Work out the finished part from the listing and answer in its coordinate system (mm). A direction names the side the tool comes from. Coordinates: 2 decimals unless noted, no trailing zeros. Loops run counter-clockwise (first coordinate to the right, second up) from the corner with the lowest first, then second, coordinate; pieces in that order, holes last. Notation, with made-up numbers: (86.25, 81.5) -> (129.25, 81.5) arc R20 ccw to (129.25, 110.5) -> close; hole circle Ø4 at (67.25, 19). An arc over 180 degrees is marked (long way). Use a Markdown table: item, result. Add a question column.
```python
from build123d import *

# Parameters (mm, degrees)
SKETCH_R     = 11.5
SKETCH_R_2   = 1.3
PAD_DEPTH    = 3
POCKET_DEPTH = 1.4


with BuildPart() as part:
    # Sketch → Pad (new body)
    with BuildSketch(Plane.XY):
        with BuildLine():
            ThreePointArc((13.066667, 5.026154), (0, 14), (-13.066667, 5.026154))
            ThreePointArc((-17.230769, 2.485461), (-14.71661, 3.047599), (-13.066667, 5.026154))
            ThreePointArc((-17.230769, 2.485461), (-20, 0), (-17.230769, -2.485461))
            ThreePointArc((-13.066667, -5.026154), (-14.71661, -3.047599), (-17.230769, -2.485461))
            ThreePointArc((-13.066667, -5.026154), (0, -14), (13.066667, -5.026154))
            ThreePointArc((17.230769, -2.485461), (14.71661, -3.047599), (13.066667, -5.026154))
            ThreePointArc((17.230769, -2.485461), (20, 0), (17.230769, 2.485461))
            ThreePointArc((13.066667, 5.026154), (14.71661, 3.047599), (17.230769, 2.485461))
        make_face()
        Circle(SKETCH_R, mode=Mode.SUBTRACT)
        with Locations((-17.5, 0)):
            Circle(SKETCH_R_2, mode=Mode.SUBTRACT)
        with Locations((17.5, 0)):
            Circle(SKETCH_R_2, mode=Mode.SUBTRACT)
    extrude(amount=PAD_DEPTH)

    # Sketch001 (on Face13 of Pad) → Pocket (cut)
    with BuildSketch(Plane.XY.offset(3)):
        with BuildLine():
            ThreePointArc((-9, -7.158911), (0, -11.5), (9, -7.158911))
            Line((10.956522, -8.715195), (9, -7.158911))
            ThreePointArc((-10.956522, -8.715195), (0, -14), (10.956522, -8.715195))
            Line((-10.956522, -8.715195), (-9, -7.158911))
        make_face()
    extrude(amount=-POCKET_DEPTH, mode=Mode.SUBTRACT)


solid = part.part
```
Item 1: Find the intervals of material crossed by probe 1 along Y at (x, z) = (17.5, 1.8); probe 2 along Y at (x, z) = (0, 1.5); probe 3 along X at (y, z) = (3.5, 0.85), in increasing order.
Item 2: Given pin 1 (2 mm diameter, centred on x = -4.5, y = -10.5, fed in from +Z), flat-ended and moving along its own axis, determine where the tip first touches the part or whether it passes through.
Item 3: Section D-D (y = 12) is taken. Determine the outline of the cut face in (x, z), then the cut area to 3 significant figures.
Item 4: Section C-C (y = -4.5) is taken. Determine the outline of the cut face in (x, z).
Item 5: Section B-B (y = 0) is taken. Determine the outline of the cut face in (x, z), then the cut area to 3 significant figures.
Item 6: For faces 4 (the face through (9.992, -7.948, 2.31)), 5 (the face through (0, -14, 1)), determine the directions among +Z, -Z, +X, -X, +Y, -Y from which every point of the face is accessible in a straight line to the end or side of a thin tool.
Item 7: Section A-A (x = 0) is taken. Determine the outline of the cut face in (y, z), then the cut area to 3 significant figures.
Item 8: For a pull along Y with two mould halves and no side action, classify faces 1 (the face through (16.2, 0.06, 1.48)), 2 (the face through (14.685, 3.067, 1.479)), 3 (the face through (-14.685, -3.067, 1.479)) as +Y half, -Y half, draft (parallel to the pull), parting line (faces both ways), or undercut.
Output:
| question | item | result |
|---|---|---|
| 1 | probe 1 | y = -2.5 to -1.3, 1.3 to 2.5 |
| 1 | probe 2 | y = -14 to -11.5, 11.5 to 14 |
| 1 | probe 3 | x = -14.11 to -10.95, 10.95 to 14.11 |
| 2 | pin 1 | stops at z = 1.6 |
| 3 | outline | (-7.21, 0) -> (7.21, 0) -> (7.21, 3) -> (-7.21, 3) -> close |
| 3 | area | 43.3 mm2 |
| 4 | outline | (-13.31, 0) -> (-10.58, 0) -> (-10.58, 3) -> (-13.31, 3) -> close; (10.58, 0) -> (13.31, 0) -> (13.31, 3) -> (10.58, 3) -> close |
| 5 | outline | (-20, 0) -> (-18.8, 0) -> (-18.8, 3) -> (-20, 3) -> close; (-16.2, 0) -> (-11.5, 0) -> (-11.5, 3) -> (-16.2, 3) -> close; (11.5, 0) -> (16.2, 0) -> (16.2, 3) -> (11.5, 3) -> close; (18.8, 0) -> (20, 0) -> (20, 3) -> (18.8, 3) -> close |
| 5 | area | 35.4 mm2 |
| 6 | face 4 | +Z, -Y |
| 6 | face 5 | +Z, -Z, -Y |
| 7 | outline | (-14, 0) -> (-11.5, 0) -> (-11.5, 1.6) -> (-14, 1.6) -> close; (11.5, 0) -> (14, 0) -> (14, 3) -> (11.5, 3) -> close |
| 7 | area | 11.5 mm2 |
| 8 | face 1 | undercut |
| 8 | face 2 | +Y half |
| 8 | face 3 | -Y half |
